```python
from build123d import *

# Parameters (mm, degrees)
F1_DEPTH = 12.7
F2_W     = 38.1
F2_H     = 6.35
F3_DEPTH = 50.8
F5_DEPTH = 25.4
F8_W     = 130.532998
F8_H     = 167.270158
F9_DEPTH = 25.4


with BuildPart() as f1:
    # F0 (on Top) → F1 (new body)
    with BuildSketch(Plane.XY):
        with BuildLine():
            Line((4.064, 127), (4.064, -127))
            Line((4.064, -127), (-4.064, -127))
            Line((-4.064, -127), (-4.064, 127))
            Line((-4.064, 127), (-42.164, 127))
            Line((-42.164, 127), (-42.164, -127))
            Line((-42.164, -127), (-42.164, -228.6))
            Line((-42.164, -228.6), (-6.35, -228.6))
            ThreePointArc((-6.35, -228.6), (0, -222.25), (6.35, -228.6))
            Line((6.35, -228.6), (42.164, -228.6))
            Line((42.164, -228.6), (42.164, -127))
            Line((42.164, -127), (42.164, 127))
            Line((42.164, 127), (4.064, 127))
        make_face()
        with BuildLine():
            Line((24.050886, -254.468208), (42.164, -228.6))
            Line((42.164, -228.6), (6.35, -228.6))
            ThreePointArc((6.35, -228.6), (0, -234.95), (-6.35, -228.6))
            Line((-6.35, -228.6), (-42.164, -228.6))
            Line((-42.164, -228.6), (-24.050886, -254.468208))
            Line((-24.050886, -254.468208), (24.050886, -254.468208))
        make_face()
    extrude(amount=F1_DEPTH)

    # F2 (on face) → F3 (join)
    with BuildSketch(Plane.XY.offset(12.7)):
        with Locations((-23.114, -123.825)):
            Rectangle(F2_W, F2_H)
    extrude(amount=F3_DEPTH)

    # F4 (on face) → F5 (cut)
    with BuildSketch(Plane.XZ.offset(127)):
        Polygon((-42.164, 12.7), (-4.064, 63.5), (-42.164, 63.5), align=None)
    extrude(amount=-F5_DEPTH, mode=Mode.SUBTRACT)

    # F6: F1 across plane


with BuildPart() as f1_1:
    add(f1.part)
    add(f1.part.mirror(Plane.YZ))

    # F7: F1 across plane


with BuildPart() as f1_2:
    add(f1_1.part)
    add(f1_1.part.mirror(Plane.XZ))

    # F8 (on face) → F9 (cut)
    with BuildSketch(Plane.XY.offset(12.7)):
        with Locations((23.102499, 210.635079)):
            Rectangle(F8_W, F8_H)
    extrude(amount=-F9_DEPTH, mode=Mode.SUBTRACT)


solid = f1_2.part
```
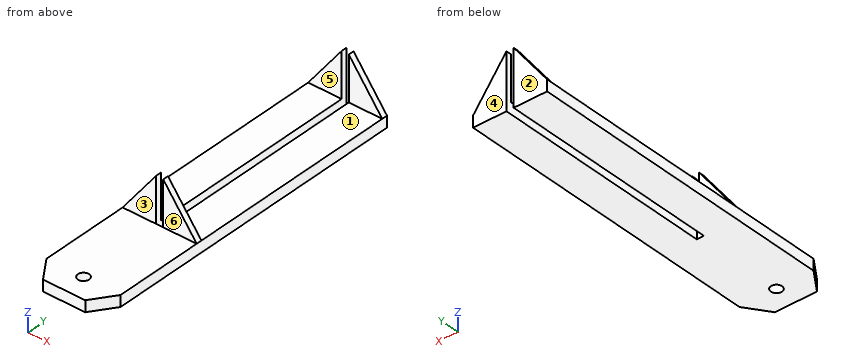
Input: part model. Units: mm. Frame: model coordinates. Face numbers are marked on the shaded views. A direction names the side the tool comes from. Give positions to 0.01 mm unless a question says otherwise; leave off trailing zeros. Order: outer loops, then holes, each group sorted by start corner. A loop starts at its lowest first (then second) coordinate and runs counter-clockwise, first axis right, second up.
1. Line query: probe 1 along X at (y, z) = (-84.5, 12); probe 2 along Y at (x, z) = (0, 9.25); probe 3 along Y at (x, z) = (7.5, 54). Output: solid intervals per line, ascending.
Computed:
probe 1: x = -42.16 to -4.06, 4.06 to 42.16
probe 2: y = -254.47 to -234.95, -222.25 to -127
probe 3: y = -127 to -120.65, 120.65 to 127
2. Set-up query: the marked faces 4, 5 and 6. Return all of +Z, -Z, +X, -X, +Y, -Y with unobstructed straight access to the full face (end or side cutting, diameter ignored); none if empty.
Computed:
face 4: +Z, -Z, +X, -X, +Y
face 5: +Z, +X, -X
face 6: +Z, +X, -X, -Y
3. Pin query (flat end, axial travel): pin 1 Ø12 at (y, z) = (-135, 25.5) entering from +X; pin 2 Ø19 at (x, y) = (-24, -58.5) entering from +Z; pin 3 Ø19 at (x, z) = (-28.5, 35.5) entering from -Y; pin 4 Ø2.5 at (x, z) = (2, 6.5) entering from +Y. Return the tip coordinate at first contact, or that it passes through.
Computed:
pin 1: passes through
pin 2: stops at z = 12.7
pin 3: stops at y = -127
pin 4: stops at y = -127
4. Cut plane B-B (y = -111.5). Return loops of the section in (x, z).
Computed:
outline: (-42.16, 0) - (-4.06, 0) - (-4.06, 12.7) - (-42.16, 12.7) - close; (4.06, 0) - (42.16, 0) - (42.16, 12.7) - (4.06, 12.7) - close
5. Draft query along Y for the marked faces 1, 2 and 3. Return one class per face: released by +Y, released by -Y, zero draft, split by the parting line, or undercut.
Computed:
face 1: undercut
face 2: released by +Y
face 3: released by -Y
6. Cut plane A-A (x = 0). Return loops of the section in (y, z).
Computed:
outline: (-254.47, 0) - (-234.95, 0) - (-234.95, 12.7) - (-254.47, 12.7) - close; (-222.25, 0) - (-127, 0) - (-127, 12.7) - (-222.25, 12.7) - close
7. Cut plane C-C (z = 51). Return loops of the section in (x, y).
Computed:
outline: (-13.44, -127) - (-4.06, -127) - (-4.06, -120.65) - (-13.44, -120.65) - close; (-13.44, 120.65) - (-4.06, 120.65) - (-4.06, 127) - (-13.44, 127) - close; (4.06, -127) - (13.44, -127) - (13.44, -120.65) - (4.06, -120.65) - close; (4.06, 120.65) - (13.44, 120.65) - (13.44, 127) - (4.06, 127) - close
8. Cut plane D-D (x = 33). Return loops of the section in (y, z), and give its area (3 significant figures).
Computed:
outline: (-241.69, 0) - (127, 0) - (127, 24.92) - (120.65, 24.92) - (120.65, 12.7) - (-120.65, 12.7) - (-120.65, 24.92) - (-127, 24.92) - (-127, 12.7) - (-241.69, 12.7) - close
area: 4,840 mm2
